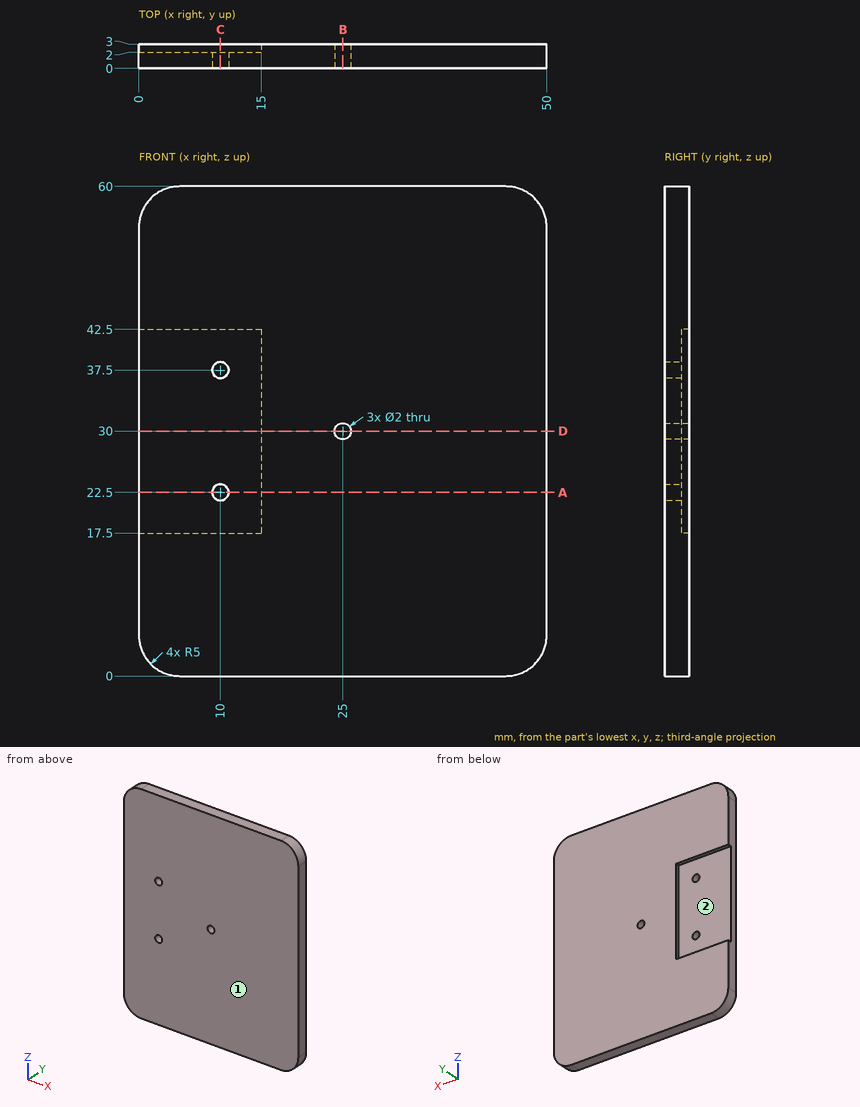
Geometry check sheet. Reference: drawing and pictorial views, mm from the part's lowest x, y, z. Round coordinates to 2 decimals unless told otherwise and drop trailing zeros. Order: outer loops, then holes, each group sorted by start corner. A loop starts at its lowest first (then second) coordinate and runs counter-clockwise, first axis right, second up. Notation, with made-up numbers: M -9.5,60.5 L 6.5,60.5 A14 ccw 6.5,64.5 Z; hole C -22,54 d5. An arc over 180 degrees is marked long. Answer in a Markdown table with one row per item.
(1) Draft check along Z on the marked faces 1 and 2. Enter one of: released by +Z, released by -Z, zero draft, split by the parting line, or undercut.
Responses:
| item | result |
|---|---|
| face 1 | zero draft |
| face 2 | undercut |
(2) Scan lines: probe 1 along Z at (x, y) = (10, 0.65); probe 2 along X at (y, z) = (1.15, 30); probe 3 along X at (y, z) = (1.3, 22.5). Record each from-to range of solid material in increasing order. Write a range as from..to.
Responses:
| item | result |
|---|---|
| probe 1 | z = 0..21.5, 23.5..36.5, 38.5..60 |
| probe 2 | x = 0..24, 26..50 |
| probe 3 | x = 0..9, 11..50 |
(3) Go/stop test with flat-tipped pins: P1, Ø1.8, axis at x = 10, z = 37.5, coming from the -Y side; P2, Ø7.5, axis at x = 5.5, z = 25.5, coming from the +Y side; P3, Ø1.1, axis at x = 4, y = 2.5, coming from the -Z side. Record where each tip stops, or that it passes through.
Responses:
| item | result |
|---|---|
| P1 | passes through |
| P2 | stops at y = 2 |
| P3 | stops at z = 0.02 |
(4) Sectioned sample at D-D, the plane z = 30. Record the cut outline in (x, y).
Responses:
| item | result |
|---|---|
| outline | M 0,0 L 24,0 L 24,3 L 15,3 L 15,2 L 0,2 Z; M 26,0 L 50,0 L 50,3 L 26,3 Z |
(5) Sectioned sample at B-B, the plane x = 25. Record the cut outline in (y, z).
Responses:
| item | result |
|---|---|
| outline | M 0,0 L 3,0 L 3,29 L 0,29 Z; M 0,31 L 3,31 L 3,60 L 0,60 Z |
(6) Sectioned sample at C-C, the plane x = 10. Record the cut outline in (y, z).
Responses:
| item | result |
|---|---|
| outline | M 0,0 L 3,0 L 3,17.5 L 2,17.5 L 2,21.5 L 0,21.5 Z; M 0,23.5 L 2,23.5 L 2,36.5 L 0,36.5 Z; M 0,38.5 L 2,38.5 L 2,42.5 L 3,42.5 L 3,60 L 0,60 Z |
(7) Sectioned sample at A-A, the plane z = 22.5. Record the cut outline in (x, y), and give its area (3 significant figures).
Responses:
| item | result |
|---|---|
| outline | M 0,0 L 9,0 L 9,2 L 0,2 Z; M 11,0 L 50,0 L 50,3 L 15,3 L 15,2 L 11,2 Z |
| area | 131 mm² |
